Design review of the part shown in the three views and the two pictorial views. Dimensions are in mm from the part's minimum x, y and z. A direction names the side the tool comes from. Round coordinates to 2 decimals unless told otherwise and drop trailing zeros. Order: outer loops, then holes, each group sorted by start corner. A loop starts at its lowest first (then second) coordinate and runs counter-clockwise, first axis right, second up.
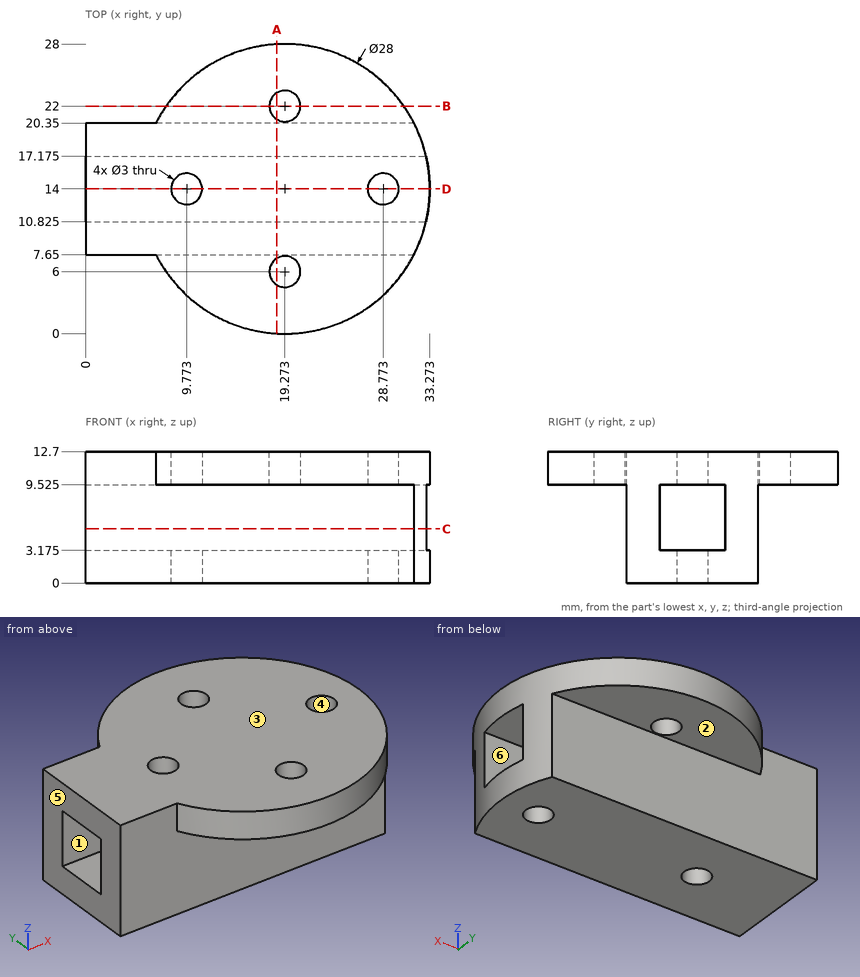
1) Take a section at D-D on y = 14. Give the boundary of the cut face in (x, z) (3 decimals).
Results:
outline: (0, 0) - (8.273, 0) - (8.273, 3.175) - (0, 3.175) - close; (0, 9.525) - (8.273, 9.525) - (8.273, 12.7) - (0, 12.7) - close; (11.273, 0) - (27.273, 0) - (27.273, 3.175) - (11.273, 3.175) - close; (11.273, 9.525) - (27.273, 9.525) - (27.273, 12.7) - (11.273, 12.7) - close; (30.273, 0) - (33.273, 0) - (33.273, 3.175) - (30.273, 3.175) - close; (30.273, 9.525) - (33.273, 9.525) - (33.273, 12.7) - (30.273, 12.7) - close
2) Take a section at A-A on x = 18.5. State how many separate pieces and enclosed holes the cut face has, plus the area to 3 significant figures.
Results:
separate pieces: 3
enclosed holes: 1
area: 153 mm2
3) Take a section at B-B on y = 22. Give the boundary of the cut face in (x, z) (3 decimals).
Results:
outline: (7.784, 9.525) - (17.773, 9.525) - (17.773, 12.7) - (7.784, 12.7) - close; (20.773, 9.525) - (30.762, 9.525) - (30.762, 12.7) - (20.773, 12.7) - close
4) The part is to be moulded in two halves that separate along X. For the marked faces 4, 5 and 6, say which applies: released by +X, released by -X, zero draft, split by the parting line, or undercut.
Results:
face 4: undercut
face 5: released by -X
face 6: zero draft
5) To check wall thickness, follow line 1 along Y through (x, z) = (9.5, 9) (3 decimals); line 2 along Z through (x, y) = (21, 13.5) (3 decimals). State the ranges of each line that lie inside material, in increasing order.
Results:
line 1: y = 7.65 to 10.825, 17.175 to 20.35
line 2: z = 0 to 3.175, 9.525 to 12.7
6) Clearance check with flat-ended pins moving along their axes: P1, Ø5, axis at y = 3.5, z = 10, coming from the -X side; P2, Ø4, axis at x = 11, z = 6.5, coming from the -Y side; P3, Ø1.9, axis at x = 23.5, z = 7.5, coming from the +Y side. State where each tip first meets the part, or that it passes through.
Results:
P1: stops at x = 7.78
P2: stops at y = 7.65
P3: stops at y = 20.35
7) For the marked faces 1, 2 and 3, list the 3-axis set-ups (+Z, -Z, +X, -X, +Y, -Y) from which the entire face can be reached by the end or side of a thin tool; tool diameter is ignored.
Results:
face 1: +X, -X
face 2: -Z, +X, -X, +Y
face 3: +Z, +X, -X, +Y, -Y
8) Take a section at C-C on z = 5.25. Give the boundary of the cut face in (x, y) (3 decimals), plus the area to 3 significant figures.
Results:
outline: (0, 7.65) - (31.75, 7.65) arc R14 ccw to (32.908, 10.825) - (0, 10.825) - close; (0, 17.175) - (32.908, 17.175) arc R14 ccw to (31.75, 20.35) - (0, 20.35) - close
area: 206 mm2
